Read the model definition and answer for the solid it produces. Units are mm, in the model's axes. Face numbers are marked on the shaded views. A direction names the side the tool comes from. Coordinates: 2 decimals unless noted, no trailing zeros. Write each loop counter-clockwise with the first axis right and the second up, starting at its lowest first coordinate (ties: lowest second). Pieces come first, ordered by that corner, then holes.
(1) Given pin 1 (21.5 mm diameter, centred on x = 0, z = 25, fed in from -Y), flat-ended and moving along its own axis, determine where the tip first touches the part or whether it passes through.
(2) Find the intervals of material crossed by probe 1 along Y at (x, z) = (-21, 20); probe 2 along X at (y, z) = (-24.45, 25), in increasing order.
(3) Section C-C on z = 9.5 is taken. Write down the section's boundary in (x, y).
(4) Section D-D on y = 4.5 is taken. Write down the section's boundary in (x, z).
(5) Which of the six approach directions +Z, -Z, +X, -X, +Y, -Y give full straight-line access (tool end or side, diameter ignored) to the marked faces 1 and 2?
(6) Section A-A on z = 40.5 is taken. Write down the section's boundary in (x, y), then the cut area to 3 significant figures.
(7) Section B-B on x = 0 is taken. Write down the section's boundary in (y, z), then the cut area to 3 significant figures.
from build123d import *

# Parameters (mm, degrees)
ESBO_O1_W                = 50
ESBO_O1_H                = 50
ESBO_O1_W_2              = 47
ESBO_O1_H_2              = 47
RESSALTO_EXTRUS_O1_DEPTH = 50
ESBO_O2_R                = 2.5
CORTE_EXTRUS_O2_DEPTH    = 10
ESBO_O3_R                = 12
CORTE_EXTRUS_O3_DEPTH    = 10
ESBO_O4_R                = 1.5
CORTE_EXTRUS_O5_DEPTH    = 10
ESBO_O5_W                = 10
ESBO_O5_H                = 36.830257898
CORTE_EXTRUS_O6_DEPTH    = 10


with BuildPart() as part:
    # Esboço1 → Ressalto-extrusão1 (new body)
    with BuildSketch(Plane.XY):
        Rectangle(ESBO_O1_W, ESBO_O1_H)
        Rectangle(ESBO_O1_W_2, ESBO_O1_H_2, mode=Mode.SUBTRACT)
    extrude(amount=RESSALTO_EXTRUS_O1_DEPTH)

    # Esboço2 → Corte-extrusão2 (cut)
    with BuildSketch(Plane(origin=(0, 25, 0), x_dir=(1, 0, 0), z_dir=(0, 1, 0))):
        with Locations((-8.838834765, -16.161165235)):
            Circle(ESBO_O2_R)
        with Locations((8.838834765, -16.161165235)):
            Circle(ESBO_O2_R)
        with Locations((-8.838834765, -33.838834765)):
            Circle(ESBO_O2_R)
        with Locations((8.838834765, -33.838834765)):
            Circle(ESBO_O2_R)
    extrude(amount=-CORTE_EXTRUS_O2_DEPTH, mode=Mode.SUBTRACT)

    # Esboço3 → Corte-extrusão3 (cut)
    with BuildSketch(Plane(origin=(0, -23.5, 0), x_dir=(1, 0, 0), z_dir=(0, 1, 0))):
        with Locations((0, -25)):
            Circle(ESBO_O3_R)
    extrude(amount=-CORTE_EXTRUS_O3_DEPTH, mode=Mode.SUBTRACT)

    # Esboço4 → Corte-extrusão5 (cut)
    with BuildSketch(Plane.XZ.offset(25)):
        with Locations((15.5, 40.5)):
            Circle(ESBO_O4_R)
        with Locations((15.5, 9.5)):
            Circle(ESBO_O4_R)
        with Locations((-15.5, 40.5)):
            Circle(ESBO_O4_R)
        with Locations((-15.5, 9.5)):
            Circle(ESBO_O4_R)
    extrude(amount=-CORTE_EXTRUS_O5_DEPTH, mode=Mode.SUBTRACT)

    # Esboço5 → Corte-extrusão6 (cut)
    with BuildSketch(Plane.XZ.offset(25)):
        with Locations((0, 50)):
            Rectangle(ESBO_O5_W, ESBO_O5_H)
    extrude(amount=-CORTE_EXTRUS_O6_DEPTH, mode=Mode.SUBTRACT)


solid = part.part
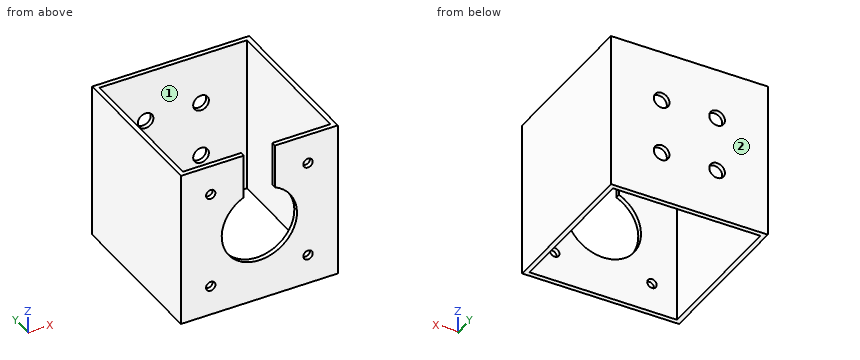
Response:
1. pin 1: stops at y = 23.5
2. probe 1: y = -25 to -23.5, 23.5 to 25
2. probe 2: x = -25 to -12, 12 to 25
3. outline: (-25, -25) - (-17, -25) - (-17, -23.5) - (-23.5, -23.5) - (-23.5, 23.5) - (23.5, 23.5) - (23.5, -23.5) - (17, -23.5) - (17, -25) - (25, -25) - (25, 25) - (-25, 25) - close; (-14, -25) - (14, -25) - (14, -23.5) - (-14, -23.5) - close
4. outline: (-25, 0) - (-23.5, 0) - (-23.5, 50) - (-25, 50) - close; (23.5, 0) - (25, 0) - (25, 50) - (23.5, 50) - close
5. face 1: +Z, -Z
5. face 2: +Z, -Z, +X, -X, +Y
6. outline: (-25, -25) - (-17, -25) - (-17, -23.5) - (-23.5, -23.5) - (-23.5, 23.5) - (23.5, 23.5) - (23.5, -23.5) - (17, -23.5) - (17, -25) - (25, -25) - (25, 25) - (-25, 25) - close; (-14, -25) - (-5, -25) - (-5, -23.5) - (-14, -23.5) - close; (5, -25) - (14, -25) - (14, -23.5) - (5, -23.5) - close
6. area: 267 mm2
7. outline: (-25, 0) - (-23.5, 0) - (-23.5, 13) - (-25, 13) - close; (23.5, 0) - (25, 0) - (25, 50) - (23.5, 50) - close
7. area: 94.5 mm2
